Here's the drawing with two shaded views (mm, measured from the low corner). I have some questions. A direction names the side the tool comes from. Coordinates: 2 decimals unless noted, no trailing zeros. Write each loop counter-clockwise with the first axis right and the second up, starting at its lowest first coordinate (ties: lowest second). Pieces come first, ordered by that corner, then holes.
Item 1: I want a section at B-B on x = 50.5. Please give me the cut outline in (y, z), then the cut area to 3 significant figures.
Item 2: I want a section at C-C on x = 40. Please give me the cut outline in (y, z).
Item 3: Which directions (+Z, -Z, +X, -X, +Y, -Y) give clear straight access to the entire face, cutting with the end or side of a thin tool? Please do the marked faces 1 and 2.
Item 4: If I drill on probe 1 along Y at (x, z) = (40, 0.9); probe 2 along Z at (x, y) = (29, 51), over which ranges is the centre line in solid material (lowest first)?
Item 5: I want a section at A-A on y = 40. Please give me the cut outline in (x, z), then the cut area to 3 significant figures.
Item 6: For P1, Ø20, axis at x = 35.5, y = 45.5, coming from the -Z side, with a flat end and sliding along its axis, tell me the tip position at first contact or that it passes through.
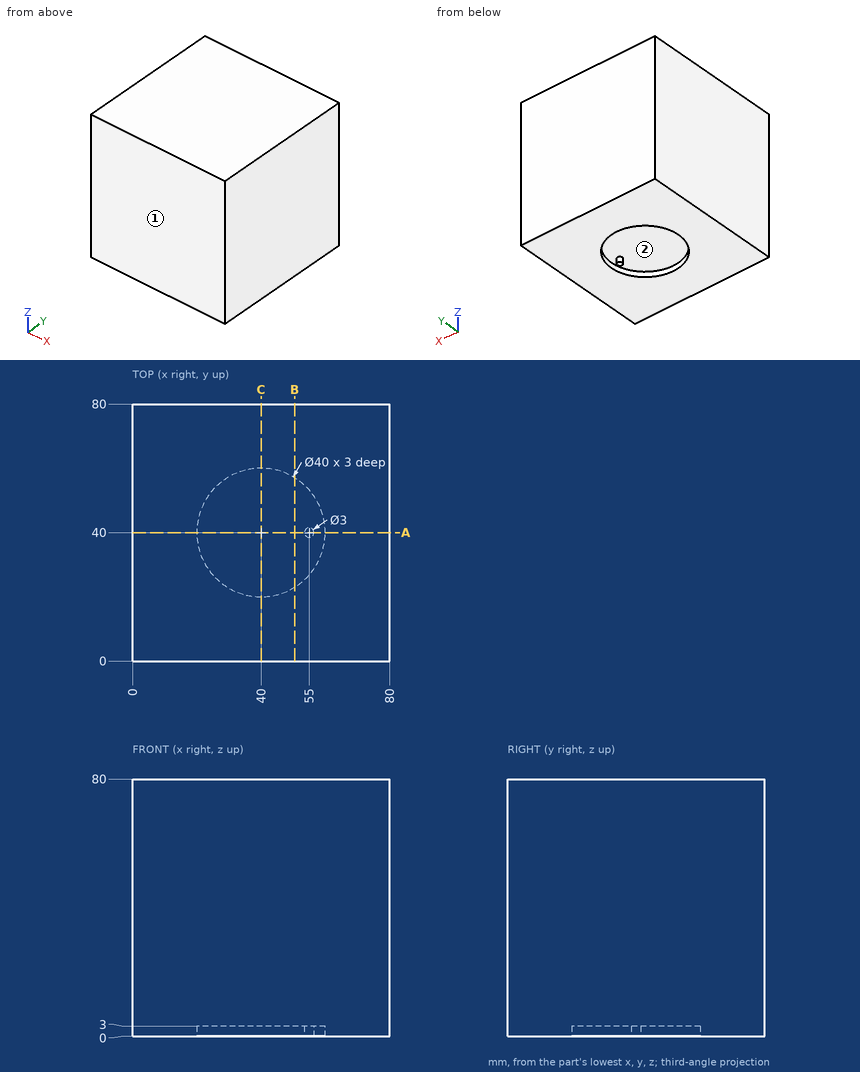
Response values:
1. outline: (0, 0) - (22.98, 0) - (22.98, 3) - (57.02, 3) - (57.02, 0) - (80, 0) - (80, 80) - (0, 80) - close
1. area: 6,300 mm2
2. outline: (0, 0) - (20, 0) - (20, 3) - (60, 3) - (60, 0) - (80, 0) - (80, 80) - (0, 80) - close
3. face 1: +Z, -Z, +X, -X, -Y
3. face 2: -Z
4. probe 1: y = 0 to 20, 60 to 80
4. probe 2: z = 3 to 80
5. outline: (0, 0) - (20, 0) - (20, 3) - (53.5, 3) - (53.5, 0) - (56.5, 0) - (56.5, 3) - (60, 3) - (60, 0) - (80, 0) - (80, 80) - (0, 80) - close
5. area: 6,290 mm2
6. P1: stops at z = 3
